Input: part model. Units: mm. Frame: model coordinates. A direction names the side the tool comes from. Give positions to 0.01 mm unless a question says otherwise; leave off trailing zeros. Write each loop counter-clockwise with the first axis right and the second up, starting at its lowest first coordinate (ties: lowest second). Pieces come first, ordered by that corner, then holes. Notation, with made-up numbers: (14.5, 14) - (71.5, 14) arc R15 cw to (71.5, 22) - close; hole circle Ø1 at (23, -4). An arc over 180 degrees is marked (long way). Use a Markdown table: item, result. Add a question column.
1. Section query A-A, the plane x = 0. Return loops of the section in (y, z).
2. Section query C-C, the plane z = 7. Return loops of the section in (x, y).
3. Set-up query: faces 1 (the flat face through (7, -9, 0)), 2 (the cylindrical face through (79, -13, 0)), 3 (the flat face through (46, -8, 8)), 4 (the flat face through (45, -8, -8)), 5 (the flat face through (77, -8.074, 0)). Return all of +Z, -Z, +X, -X, +Y, -Y with unobstructed straight access to the full face (end or side cutting, diameter ignored); none if empty.
4. Mould query, pull axis X, two halves, no side actions, for faces 6 (the flat face through (41.79, -12.98, 0.11)), 7 (the flat face through (7, 0, 0)), 8 (the cylindrical face through (-6, -4, 0)). Classes: released by +X, released by -X, zero draft, split by the parting line, or undercut.
5. Pin query (flat end, axial travel): pin 1 (7.5 mm diameter, centred on x = -1, z = 5.5, fed in from -Y); pin 2 (3 mm diameter, centred on x = 3, y = -3, fed in from -Z); pin 3 (3 mm diameter, centred on x = 22, y = -5, fed in from -Z); pin 4 (10 mm diameter, centred on y = -8, z = 0.5, fed in from -X). Return the tip coordinate at first contact, or that it passes through.
6. Material intervals for probe 1 along Z at (x, y) = (85, -12.75); probe 2 along Z at (x, y) = (0, -4); probe 3 along Y at (x, z) = (8, -4.75), sorted ascending.
7. Section query D-D, the plane x = 85. Return loops of the section in (y, z).
8. Section query B-B, the plane y = -5.25. Return loops of the section in (x, z), plus the area to 3 significant figures.
```python
from build123d import *

# Parameters (mm, degrees)
F0_R     = 6
F1_DEPTH = 25
F3_DEPTH = 12.5
F4_R     = 15


with BuildPart() as f1:
    # F0 (on Front) → F1 (new body)
    with BuildSketch(Plane.XZ):
        with BuildLine():
            ThreePointArc((9.604686, -8), (11.753905, -4.253905), (12.5, 0))
            ThreePointArc((12.5, 0), (11.753905, 4.253905), (9.604686, 8))
            ThreePointArc((9.604686, 8), (-12.5, 0), (9.604686, -8))
        make_face()
        Circle(F0_R, mode=Mode.SUBTRACT)
        with BuildLine():
            ThreePointArc((9.604686, 8), (11.753905, 4.253905), (12.5, 0))
            ThreePointArc((12.5, 0), (11.753905, -4.253905), (9.604686, -8))
            Line((9.604686, -8), (79, -8))
            ThreePointArc((79, -8), (75, 0), (79, 8))
            Line((79, 8), (9.604686, 8))
        make_face()
        with BuildLine():
            ThreePointArc((95, 0), (89.472136, 8.944272), (79, 8))
            ThreePointArc((79, 8), (75, 0), (79, -8))
            ThreePointArc((79, -8), (89.472136, -8.944272), (95, 0))
        make_face()
        with Locations((85, 0)):
            Circle(F0_R, mode=Mode.SUBTRACT)
    extrude(amount=F1_DEPTH)

    # F2 (on Top) → F3 (intersect, symmetric)
    with BuildSketch(Plane.XY):
        Polygon((95, -17.073554), (95, -8.073554), (65.787398, -8.073554), (20, 0), (-12.5, 0), (-12.5, -9), (19.212602, -9), (65, -17.073554), align=None)
    extrude(amount=F3_DEPTH, both=True, mode=Mode.INTERSECT)

    # F4
    f4_edges = [f1.edges().sort_by_distance(p)[0] for p in [
        (79, -12.573554, -8),
        (9.604686, -4.5, -8),
        (9.604686, -4.5, 8),
        (79, -12.573554, 8),
    ]]
    fillet(f4_edges, radius=F4_R)


solid = f1.part
```
Result sheet:
| question | item | result |
|---|---|---|
| 1 | outline | (-9, -12.5) - (0, -12.5) - (0, -6) - (-9, -6) - close; (-9, 6) - (0, 6) - (0, 12.5) - (-9, 12.5) - close |
| 2 | outline | (-10.36, -9) - (19.21, -9) - (65, -17.07) - (92.14, -17.07) - (92.14, -8.07) - (65.79, -8.07) - (20, 0) - (-10.36, 0) - close |
| 3 | face 1 | +Z, -Z, -X, -Y |
| 3 | face 2 | +Y, -Y |
| 3 | face 3 | +Z, +Y, -Y |
| 3 | face 4 | -Z, +Y, -Y |
| 3 | face 5 | +Z, -Z, +X, +Y |
| 4 | face 6 | released by -X |
| 4 | face 7 | zero draft |
| 4 | face 8 | undercut |
| 5 | pin 1 | stops at y = -9 |
| 5 | pin 2 | stops at z = -12.41 |
| 5 | pin 3 | stops at z = -8 |
| 5 | pin 4 | stops at x = -12.5 |
| 6 | probe 1 | z = -10 to -6, 6 to 10 |
| 6 | probe 2 | z = -12.5 to -6, 6 to 12.5 |
| 6 | probe 3 | y = -9 to 0 |
| 7 | outline | (-17.07, -10) - (-8.07, -10) - (-8.07, -6) - (-17.07, -6) - close; (-17.07, 6) - (-8.07, 6) - (-8.07, 10) - (-17.07, 10) - close |
| 8 | outline | (6.85, -10.45) arc R15 cw to (15.07, -8) - (49.77, -8) - (49.77, 8) - (15.07, 8) arc R15 cw to (6.85, 10.45) arc R12.5 ccw (long way) to start; hole circle Ø12 at (0, 0) |
| 8 | area | 994 mm² |
